```python
from build123d import *

# Parameters (mm, degrees)
SKETCH2_W                = 14.162138344
SKETCH2_H                = 3.4
SKETCH2_W_2              = 7.073181434
SKETCH2_H_2              = 3.44
SKETCH2_R                = 0.75
SKETCH2_W_3              = 7.08895691
BOSS_EXTRUDE1_DEPTH      = 20
BOSS_EXTRUDE2_START      = -11
BOSS_EXTRUDE2_DEPTH      = 23
CUT_EXTRUDE1_DEPTH       = 23
BOSS_EXTRUDE3_DEPTH      = 20
SKETCH8_R                = 1.6
CUT_EXTRUDE2_DEPTH       = 50
CUT_EXTRUDE3_START       = 9
SKETCH9_W                = 15
SKETCH9_H                = 3
CUT_EXTRUDE3_DEPTH       = 50
SKETCH10_W               = 8
SKETCH10_H               = 3.4
BOSS_EXTRUDE4_DEPTH      = 20
CUT_EXTRUDE4_DEPTH       = 15
CUT_EXTRUDE6_DEPTH       = 15
CUT_EXTRUDE7_DEPTH       = 14.77685015
CUT_EXTRUDE7_DEPTH_BACK  = 26.48895691
CUT_EXTRUDE8_DEPTH       = 11.48895691
CUT_EXTRUDE8_DEPTH_BACK  = 11.48895691
CUT_EXTRUDE9_DEPTH       = 11.48895691
CUT_EXTRUDE9_DEPTH_BACK  = 11.48895691
SKETCH16_W               = 14.162138344
SKETCH16_H               = 9.377104558
CUT_EXTRUDE10_DEPTH      = 16.0000001
CUT_EXTRUDE10_DEPTH_BACK = 15.024346574
BOSS_EXTRUDE5_DEPTH      = 15
SKETCH18_W               = 14.162138344
SKETCH18_H               = 2
BOSS_EXTRUDE6_DEPTH      = 15
SKETCH19_W               = 15
SKETCH19_H               = 3
BOSS_EXTRUDE7_DEPTH      = 15
CUT_EXTRUDE11_DEPTH      = 11.48895691
CUT_EXTRUDE11_DEPTH_BACK = 11.48895691
SKETCH21_R               = 1.55
CUT_EXTRUDE12_DEPTH      = 20
SKETCH23_W               = 14.162138344
SKETCH23_H               = 12.378444436
CUT_EXTRUDE13_DEPTH      = 16
CUT_EXTRUDE13_DEPTH_BACK = 15.024346574
SKETCH24_W               = 14.162138344
SKETCH24_H               = 2.5
BOSS_EXTRUDE8_DEPTH      = 5
CUT_EXTRUDE14_START      = -10
SKETCH25_R               = 1.55
CUT_EXTRUDE14_DEPTH      = 20


with BuildPart() as part:
    # Sketch2 → Boss-Extrude1 (new body)
    with BuildSketch(Plane.XY):
        with BuildLine():
            Line((-10.48895691, 0), (-10.48895691, -15))
            ThreePointArc((-10.48895691, -15), (0, -25.48895691), (10.48895691, -15))
            Line((10.48895691, -15), (10.48895691, 0))
            ThreePointArc((10.48895691, 0), (0, 10.48895691), (-10.48895691, 0))
        make_face()
        with BuildLine():
            ThreePointArc((-7.073181434, -14.546841059), (0.007887738, -21.627910231), (7.08895691, -14.546841059))
            Line((7.08895691, -14.546841059), (7.08895691, -0.433251968))
            ThreePointArc((7.08895691, -0.433251968), (0.007887738, 6.647817204), (-7.073181434, -0.433251968))
            Line((-7.073181434, -0.433251968), (-7.073181434, -14.546841059))
        make_face(mode=Mode.SUBTRACT)
        with Locations((0.007887738, -4.477329194)):
            Rectangle(SKETCH2_W, SKETCH2_H)
        with Locations((-3.536590717, -12.826841059)):
            Rectangle(SKETCH2_W_2, SKETCH2_H_2)
        with Locations((-3.845252141, -12.837457066)):
            Circle(SKETCH2_R, mode=Mode.SUBTRACT)
        with Locations((3.544478455, -12.826841059)):
            Rectangle(SKETCH2_W_3, SKETCH2_H_2)
        with Locations((3.845252141, -12.837457066)):
            Circle(SKETCH2_R, mode=Mode.SUBTRACT)
    extrude(amount=BOSS_EXTRUDE1_DEPTH)



with BuildPart() as body_2:
    # Sketch5 → Boss-Extrude2 (new body)
    with BuildSketch(Plane(origin=(0, 0, 0), x_dir=(0, 0, -1), z_dir=(1, 0, 0)).offset(BOSS_EXTRUDE2_START)):
        Polygon((-20, 10.48895691), (-20, 13.77685015), (0, 10.48895691), align=None)
    extrude(amount=BOSS_EXTRUDE2_DEPTH)

    # Sketch6 → Cut-Extrude1 (cut)
    with BuildSketch(Plane.XY):
        Polygon((-10.48895691, 0), (-10.48895691, 15.860273687), (-12.486191968, 15.860273687), (-12.486191968, -0.695838208), align=None)
        Polygon((10.48895691, 0), (10.48895691, 17.140856928), (14.451791198, 17.140856928), (14.085910272, 0), align=None)
    extrude(amount=CUT_EXTRUDE1_DEPTH, mode=Mode.SUBTRACT)


with BuildPart() as part_1:
    add(part.part)

    add(body_2.part)  # Boss-Extrude3 merges body 2
    # Sketch7 → Boss-Extrude3 (add)
    with BuildSketch(Plane.XY):
        Polygon((-10.48895691, 10.48895691), (-10.48895691, 0), (-4.00693271, 9.117877526), (3.3932631, 9.117877526), (10.48895691, 0), (10.48895691, 10.48895691), align=None)
    extrude(amount=BOSS_EXTRUDE3_DEPTH)

    # Sketch8 → Cut-Extrude2 (cut)
    with BuildSketch(Plane(origin=(0, 0, 0), x_dir=(1, 0, 0), z_dir=(0, 1, 0))):
        with Locations((0, -11.795956347)):
            Circle(SKETCH8_R)
    extrude(amount=CUT_EXTRUDE2_DEPTH, mode=Mode.SUBTRACT)

    # Sketch9 → Cut-Extrude3 (cut)
    with BuildSketch(Plane.XY.offset(CUT_EXTRUDE3_START)):
        with Locations((0, 8.87685015)):
            Rectangle(SKETCH9_W, SKETCH9_H)
    extrude(amount=CUT_EXTRUDE3_DEPTH, mode=Mode.SUBTRACT)

    # Sketch10 → Boss-Extrude4 (add)
    with BuildSketch(Plane.XY):
        with Locations((0, -4.477329194)):
            Rectangle(SKETCH10_W, SKETCH10_H)
    extrude(amount=-BOSS_EXTRUDE4_DEPTH)

    # Sketch11 → Cut-Extrude4 (cut)
    with BuildSketch(Plane(origin=(0, 0, 0), x_dir=(1, 0, 0), z_dir=(0, 1, 0))):
        with BuildLine():
            ThreePointArc((4, 27.93345462), (0, 23.93345462), (-4, 27.93345462))
            Line((-4, 27.93345462), (-5.669072563, 15.992564213))
            Line((-5.669072563, 15.992564213), (5.557395145, 15.474390906))
            Line((5.557395145, 15.474390906), (4, 27.93345462))
        make_face()
    extrude(amount=-CUT_EXTRUDE4_DEPTH, mode=Mode.SUBTRACT)

    # Sketch12 → Cut-Extrude6 (cut)
    with BuildSketch(Plane(origin=(0, 0, 0), x_dir=(1, 0, 0), z_dir=(0, 1, 0))):
        with BuildLine():
            ThreePointArc((-1.5, 10), (0, 8.5), (1.5, 10))
            ThreePointArc((1.5, 10), (1.499895352, 10.017718186), (1.499581421, 10.0354339))
            Line((1.499581421, 10.0354339), (-1.499581421, 10.0354339))
            ThreePointArc((-1.499581421, 10.0354339), (-1.499895352, 10.017718186), (-1.5, 10))
        make_face()
        with BuildLine():
            Line((-1.499581421, 10.0354339), (1.499581421, 10.0354339))
            ThreePointArc((1.499581421, 10.0354339), (0, 11.5), (-1.499581421, 10.0354339))
        make_face()
        with BuildLine():
            Line((-1.5, 0), (1.5, 0))
            Line((1.5, 0), (1.5, 10))
            ThreePointArc((1.5, 10), (0, 8.5), (-1.5, 10))
            Line((-1.5, 10), (-1.5, 0))
        make_face()
    extrude(amount=-CUT_EXTRUDE6_DEPTH, mode=Mode.SUBTRACT)

    # Sketch13 → Cut-Extrude7 (cut, two sides)
    with BuildSketch(Plane(origin=(0, 0, 0), x_dir=(1, 0, 0), z_dir=(0, 1, 0))) as cut_extrude7_sk:
        with BuildLine():
            Line((-7.439128098, 19.178498244), (-4, 10.024346574))
            ThreePointArc((-4, 10.024346574), (0, 14.024346574), (4, 10.024346574))
            Line((4, 10.024346574), (9.668085042, 17.513702334))
            Line((9.668085042, 17.513702334), (-7.439128098, 19.178498244))
        make_face()
    extrude(amount=CUT_EXTRUDE7_DEPTH, mode=Mode.SUBTRACT)
    extrude(cut_extrude7_sk.sketch, amount=-CUT_EXTRUDE7_DEPTH_BACK, mode=Mode.SUBTRACT)

    # Sketch14 → Cut-Extrude8 (cut, two sides)
    with BuildSketch(Plane(origin=(0, 0, 0), x_dir=(0, 0, -1), z_dir=(1, 0, 0))) as cut_extrude8_sk:
        Polygon((-26.730054166, 15.422520577), (-23.0368577, -28.4462079), (-15, -25.48895691), (-15, 13.72392169), align=None)
    extrude(amount=CUT_EXTRUDE8_DEPTH, mode=Mode.SUBTRACT)
    extrude(cut_extrude8_sk.sketch, amount=-CUT_EXTRUDE8_DEPTH_BACK, mode=Mode.SUBTRACT)

    # Sketch15 → Cut-Extrude9 (cut, two sides)
    with BuildSketch(Plane(origin=(0, 0, 0), x_dir=(0, 0, -1), z_dir=(1, 0, 0))) as cut_extrude9_sk:
        Polygon((-15, 12.95487684), (0, 7.573497647), (5.521522654, 8.824312447), (5.521522654, 13.501272135), (-15.144113177, 13.990721405), align=None)
    extrude(amount=CUT_EXTRUDE9_DEPTH, mode=Mode.SUBTRACT)
    extrude(cut_extrude9_sk.sketch, amount=-CUT_EXTRUDE9_DEPTH_BACK, mode=Mode.SUBTRACT)

    # Sketch16 → Cut-Extrude10 (cut, two sides)
    with BuildSketch(Plane.XY) as cut_extrude10_sk:
        with Locations((0.007887738, 1.911223085)):
            Rectangle(SKETCH16_W, SKETCH16_H)
    extrude(amount=CUT_EXTRUDE10_DEPTH, mode=Mode.SUBTRACT)
    extrude(cut_extrude10_sk.sketch, amount=-CUT_EXTRUDE10_DEPTH_BACK, mode=Mode.SUBTRACT)

    # Sketch17 → Boss-Extrude5 (add, through all)
    with BuildSketch(Plane.XY):
        Polygon((-7.073181434, 6.271603377), (7.08895691, 6.271603377), (7.08895691, 6.934816107), (-7.073181434, 6.934816107), (-7.073181434, 6.599775364), (-7.073181434, 6.43568937), align=None)
    extrude(amount=BOSS_EXTRUDE5_DEPTH)

    # Sketch18 → Boss-Extrude6 (add, through all)
    with BuildSketch(Plane.XY):
        with Locations((0.007887738, 2.271603377)):
            Rectangle(SKETCH18_W, SKETCH18_H)
    extrude(amount=BOSS_EXTRUDE6_DEPTH)

    # Sketch19 → Boss-Extrude7 (add)
    with BuildSketch(Plane.XY):
        with Locations((0, 8.87685015)):
            Rectangle(SKETCH19_W, SKETCH19_H)
    extrude(amount=BOSS_EXTRUDE7_DEPTH)

    # Sketch20 → Cut-Extrude11 (cut, two sides)
    with BuildSketch(Plane(origin=(0, 0, 0), x_dir=(0, 0, -1), z_dir=(1, 0, 0))) as cut_extrude11_sk:
        Polygon((-15, 12.95487684), (0, 7.573497647), (2.534300376, 12.95487684), align=None)
    extrude(amount=CUT_EXTRUDE11_DEPTH, mode=Mode.SUBTRACT)
    extrude(cut_extrude11_sk.sketch, amount=-CUT_EXTRUDE11_DEPTH_BACK, mode=Mode.SUBTRACT)

    # Sketch21 → Cut-Extrude12 (cut)
    with BuildSketch(Plane(origin=(0, 0, 0), x_dir=(1, 0, 0), z_dir=(0, 1, 0))):
        with Locations((0, -11.805650833)):
            Circle(SKETCH21_R)
    extrude(amount=CUT_EXTRUDE12_DEPTH, mode=Mode.SUBTRACT)

    # Sketch23 → Cut-Extrude13 (cut, two sides)
    with BuildSketch(Plane.XY) as cut_extrude13_sk:
        with Locations((0.007887738, -4.917618841)):
            Rectangle(SKETCH23_W, SKETCH23_H)
    extrude(amount=CUT_EXTRUDE13_DEPTH, mode=Mode.SUBTRACT)
    extrude(cut_extrude13_sk.sketch, amount=-CUT_EXTRUDE13_DEPTH_BACK, mode=Mode.SUBTRACT)

    # Sketch24 → Boss-Extrude8 (add)
    with BuildSketch(Plane.XY):
        with Locations((0.007887738, -2.978396623)):
            Rectangle(SKETCH24_W, SKETCH24_H)
    extrude(amount=BOSS_EXTRUDE8_DEPTH)

    # Sketch25 → Cut-Extrude14 (cut)
    with BuildSketch(Plane(origin=(0, 0, 0), x_dir=(1, 0, 0), z_dir=(0, 1, 0)).offset(CUT_EXTRUDE14_START)):
        with Locations((0, -2.191424263)):
            Circle(SKETCH25_R)
    extrude(amount=CUT_EXTRUDE14_DEPTH, mode=Mode.SUBTRACT)


solid = part_1.part
```
Here's how the part is built. I have some questions about the finished solid (model axes, mm). A direction names the side the tool comes from. Round coordinates to 2 decimals unless told otherwise and drop trailing zeros. Loops run counter-clockwise (first coordinate to the right, second up) from the corner with the lowest first, then second, coordinate; pieces in that order, holes last. Notation, with made-up numbers: (-33, 60.25) -> (3, 60.25) arc R23 ccw to (3, 73.25) -> close; hole circle Ø4 at (-27.75, 46). An arc over 180 degrees is marked (long way). Answer as CSV lines item,"result".
1. If we section it at A-A on y = 4: Please give me the cut outline in (x, z), plus the area to 3 significant figures.
Final values:
outline,"(-10.49, 0) -> (-7.07, 0) -> (-7.07, 15) -> (-10.49, 15) -> close; (7.09, 0) -> (10.49, 0) -> (10.49, 15) -> (7.09, 15) -> close"
area,"102 mm^2"
2. If we section it at D-D on z = 6: Please give me the cut outline in (x, y).
Final values:
outline,"(-10.49, -15) arc R10.49 ccw to (10.49, -15) -> (10.49, 9.73) -> (-10.49, 9.73) -> close; hole (-7.07, -14.55) arc R7.08 ccw to (7.09, -14.55) -> close; hole (-7.07, -11.11) -> (7.09, -11.11) -> (7.09, 1.27) -> (-7.07, 1.27) -> close; hole (-7.07, 3.27) -> (7.09, 3.27) -> (7.09, 6.27) -> (-7.07, 6.27) -> close; hole circle Ø1.5 at (-3.85, -12.84); hole circle Ø1.5 at (3.85, -12.84)"
3. If I drill on L1, parallel to Z at x = 0, y = 6.75; L2, parallel to X at y = -4.5, z = 4.75; L3, parallel to Y at x = -1.5, z = 6.25, over which ranges is the centre line in solid material (lowest first)?
Final values:
L1,"z = 0 to 0.64, 3.74 to 10.26, 13.36 to 15"
L2,"x = -10.49 to -7.07, 7.09 to 10.49"
L3,"y = -25.38 to -21.47, -14.55 to -11.11, 1.27 to 3.27, 6.27 to 9.82"
4. For pin 1 (5 mm diameter, centred on x = 0.5, y = -10.5, fed in from -Z); pin 2 (8 mm diameter, centred on x = 5, z = 6.5, fed in from +Y); pin 3 (1.2 mm diameter, centred on x = -3.85, y = -12.84, fed in from -Z); pin 4 (1 mm diameter, centred on x = 0, z = 12.5, fed in from +Y), each with a flat end and sliding along its axis, tell me the tip position at first contact or that it passes through.
Final values:
pin 1,"stops at z = 0"
pin 2,"stops at y = 11.34"
pin 3,"passes through"
pin 4,"stops at y = -11.11"
5. Which directions (+Z, -Z, +X, -X, +Y, -Y) give clear straight access to the entire face, cutting with the end or side of a thin tool? Please do faces 1 (the face through (-7.073, 5, 7)), 2 (the face through (7.089, -5, 7)), 3 (the face through (0.833, 2.258, 10.499)).
Final values:
face 1,"+Z, -Z"
face 2,"+Z"
face 3,"+Y"
6. Thinking about a two-plate mould opening in Z: for faces 4 (the face through (0.833, 8.856, 10.499)), 5 (the face through (-2, -4.228, 2)), 6 (the face through (0.833, 6.599, 10.499)), 7 (the face through (0.1, 10.3, 7.6)), which applies, released by +Z, released by -Z, zero draft, split by the parting line, or undercut?
Final values:
face 4,"undercut"
face 5,"zero draft"
face 6,"undercut"
face 7,"released by -Z"
7. If we section it at C-C on z = 1.5: Count the separate pieces of the cut face and the enclosed holes in it, plus the area to 3 significant figures.
Final values:
separate pieces,"1"
enclosed holes,"3"
area,"375 mm^2"
8. If we section it at B-B on x = 2.5: Please give me the cut outline in (y, z), plus the area to 3 significant figures.
Final values:
outline,"(-25.19, 0) -> (-21.17, 0) -> (-21.17, 15) -> (-25.19, 15) -> close; (-14.55, 0) -> (-11.11, 0) -> (-11.11, 15) -> (-14.55, 15) -> close; (-4.23, 0) -> (-1.73, 0) -> (-1.73, 5) -> (-4.23, 5) -> close; (1.27, 0) -> (3.27, 0) -> (3.27, 15) -> (1.27, 15) -> close; (6.27, 0) -> (7.57, 0) -> (12.95, 15) -> (6.27, 15) -> close"
area,"214 mm^2"
